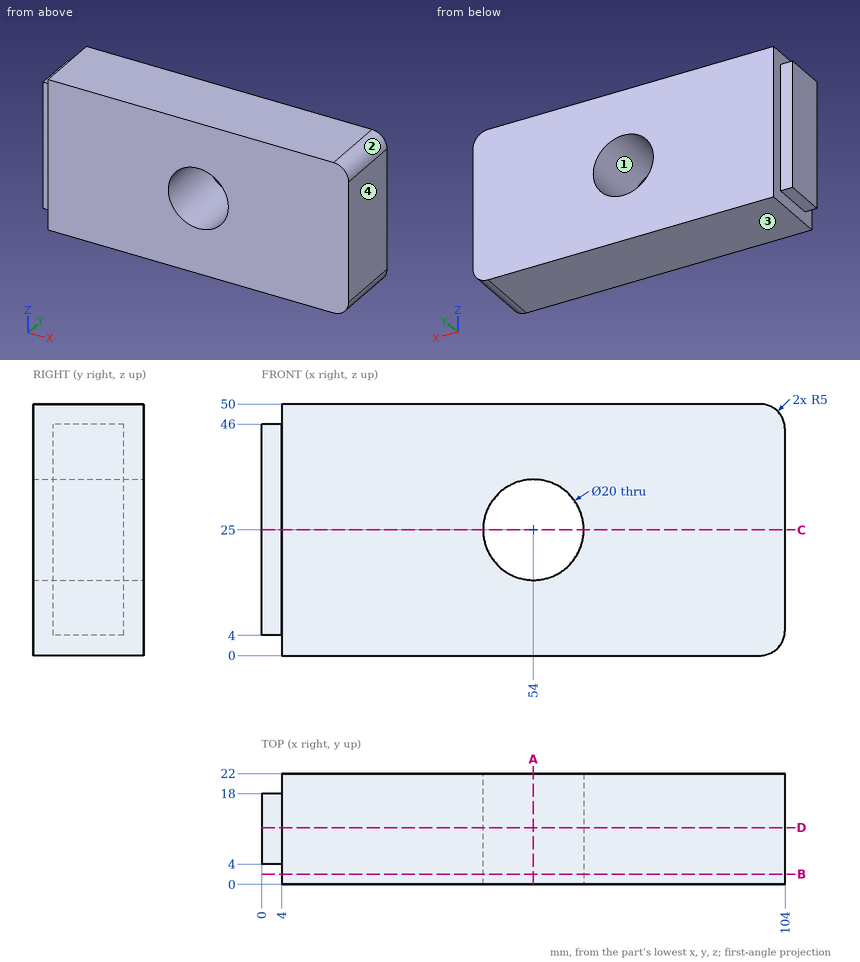
Drawing for the job (mm, zero at the part's lowest x, y, z). Coordinates: 2 decimals unless noted, no trailing zeros. Write each loop counter-clockwise with the first axis right and the second up, starting at its lowest first coordinate (ties: lowest second). Pieces come first, ordered by that corner, then holes. Notation, with made-up numbers: (62.5, -2.75) - (67.5, -2.75) arc R19 ccw to (67.5, 1.25) - close; hole circle Ø3 at (-26, -6). An arc over 180 degrees is marked (long way). Write each question's results on one line, items separated by ' | '. Start each with the question number.
1) Cut at C-C (z = 25). Write the cut outline in (x, y).
2) Flat gauge pins, fed straight in: P1, Ø3, axis at x = 1.5, z = 14.5, coming from the +Y side; P2, Ø1.2, axis at x = 2.5, z = 32.5, coming from the -Y side; P3, Ø4.5, axis at x = 1, y = 10, coming from the +Z side. Where does each tip first touch, or does it go through?
3) Cut at A-A (x = 54). Write the cut outline in (y, z), then the cut area to 3 significant figures.
4) Cut at B-B (y = 2). Write the cut outline in (x, z), then the cut area to 3 significant figures.
5) Cut at D-D (y = 11.25). Write the cut outline in (x, z), then the cut area to 3 significant figures.
6) Probe line 1 along Z through (x, y) = (54, 5.25); line 2 along X through (y, z) = (5.75, 24.5); line 3 along X through (y, z) = (18.5, 7.5). List the from-to ranges inside material, lowest first. Write a range as from..to.
7) Mould opens along Z. For the marked faces 1, 2, 3 and 4 say: pulls with the +Z half, pulls with the -Z half, needs draft (parallel to the pull), parting line crosses it, or undercut.
Returned:
1) outline: (0, 4) - (4, 4) - (4, 0) - (44, 0) - (44, 22) - (4, 22) - (4, 18) - (0, 18) - close; (64, 0) - (104, 0) - (104, 22) - (64, 22) - close
2) P1: y = 18 | P2: y = 4 | P3: z = 46
3) outline: (0, 0) - (22, 0) - (22, 15) - (0, 15) - close; (0, 35) - (22, 35) - (22, 50) - (0, 50) - close | area: 660 mm^2
4) outline: (4, 0) - (99, 0) arc R5 ccw to (104, 5) - (104, 45) arc R5 ccw to (99, 50) - (4, 50) - close; hole circle Ø20 at (54, 25) | area: 4,680 mm^2
5) outline: (0, 4) - (4, 4) - (4, 0) - (99, 0) arc R5 ccw to (104, 5) - (104, 45) arc R5 ccw to (99, 50) - (4, 50) - (4, 46) - (0, 46) - close; hole circle Ø20 at (54, 25) | area: 4,840 mm^2
6) line 1: 0..15, 35..50 | line 2: 0..44.01, 63.99..104 | line 3: 4..104
7) face 1: undercut | face 2: pulls with the +Z half | face 3: pulls with the -Z half | face 4: needs draft
